Geometry: final body of the model. Coordinates: model frame, mm. Face numbers are marked on the shaded views. Round coordinates to 2 decimals unless told otherwise and drop trailing zeros. Write each loop counter-clockwise with the first axis right and the second up, starting at its lowest first coordinate (ties: lowest second). Pieces come first, ordered by that corner, then holes. Notation, with made-up numbers: M 78,62 L 104,62 A23 cw 104,75 Z; hole C -0.5,-9 d8. An arc over 180 degrees is marked long. Use one line per item in the form item = value. Start each with the question number.
from build123d import *

# Parameters (mm, degrees)
F2_R     = 4.760298
F3_DEPTH = 9.525
F4_R     = 1.578177
F5_DEPTH = 22.225


with BuildPart() as f1:
    # F0 (on Front) → F1 (revolve)
    with BuildSketch(Plane.XZ):
        with BuildLine():
            Line((0, 38.964737), (0, -24.535263))
            Line((0, -24.535263), (4.922395, -24.535263))
            Line((4.922395, -24.535263), (7.092721, -20.039586))
            Line((7.092721, -20.039586), (7.092721, -9.498))
            ThreePointArc((7.092721, -9.498), (15.409558, -6.117437), (23.523532, -9.959494))
            ThreePointArc((23.523532, -9.959494), (31.75, 0.193678), (24.824452, 11.275126))
            ThreePointArc((24.824452, 11.275126), (20.770385, 7.146589), (15.368029, 5.074192))
            ThreePointArc((15.368029, 5.074192), (9.67931, 6.104722), (7.092721, 11.275126))
            Line((7.092721, 11.275126), (7.092721, 38.964737))
            Line((7.092721, 38.964737), (0, 38.964737))
        make_face()
    revolve(axis=Axis((0, 0, 7.214737), (0, 0, 1)))

    # F2 (on face) → F3 (cut)
    with BuildSketch(Plane.XY.offset(38.964737)):
        Circle(F2_R)
    extrude(amount=-F3_DEPTH, mode=Mode.SUBTRACT)

    # F4 (on face) → F5 (cut)
    with BuildSketch(Plane(origin=(0, 0, -24.535263), x_dir=(1, 0, 0), z_dir=(0, 0, -1))):
        Circle(F4_R)
    extrude(amount=-F5_DEPTH, mode=Mode.SUBTRACT)


solid = f1.part
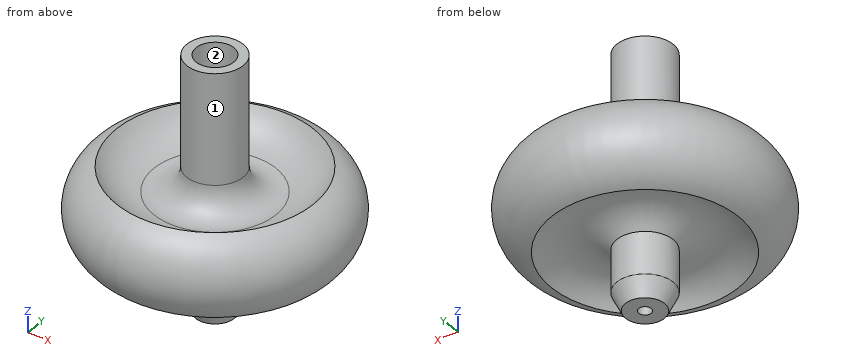
1. Ray query, probe 1 along Y at (x, z) = (-5.5, 11); probe 2 along X at (y, z) = (-2.5, -7.5); probe 3 along Y at (x, z) = (0, -19.5). Return the intervals inside material, ascending.
2. Pull-direction query (X, two-part tool) for the marked faces 1 and 2; classes: released by +X, released by -X, zero draft, split by the parting line, or undercut.
3. Contact query for flat-ended pins moving along their axis: pin 1 (1.5 mm diameter, centred on x = 6, y = -11.5, fed in from +Z); pin 2 (5 mm diameter, centred on y = 9.5, z = 4, fed in from -X); pin 3 (8 mm diameter, centred on x = -8.5, y = -9.5, fed in from +Z). Output: stop coordinate, or through.
4. Section query A-A (z = 30.5). Return loops of the section in (x, y).
5. Section query B-B (z = -3.5). Return loops of the section in (x, y).
Checks:
q1.probe_1 = -24.84 to -24.02, -4.49 to 4.49, 24.02 to 24.84
q1.probe_2 = -27.91 to -20.33, -9.38 to 9.38, 20.33 to 27.91
q1.probe_3 = -7.09 to -1.58, 1.58 to 7.09
q2.face_1 = split by the parting line
q2.face_2 = undercut
q3.pin_1 = 4.95
q3.pin_2 = -30.75
q3.pin_3 = 6.96
q4.outline = C 0,0 d14.19; hole C 0,0 d9.52
q5.outline = C 0,0 d61.77; hole C 0,0 d3.16
